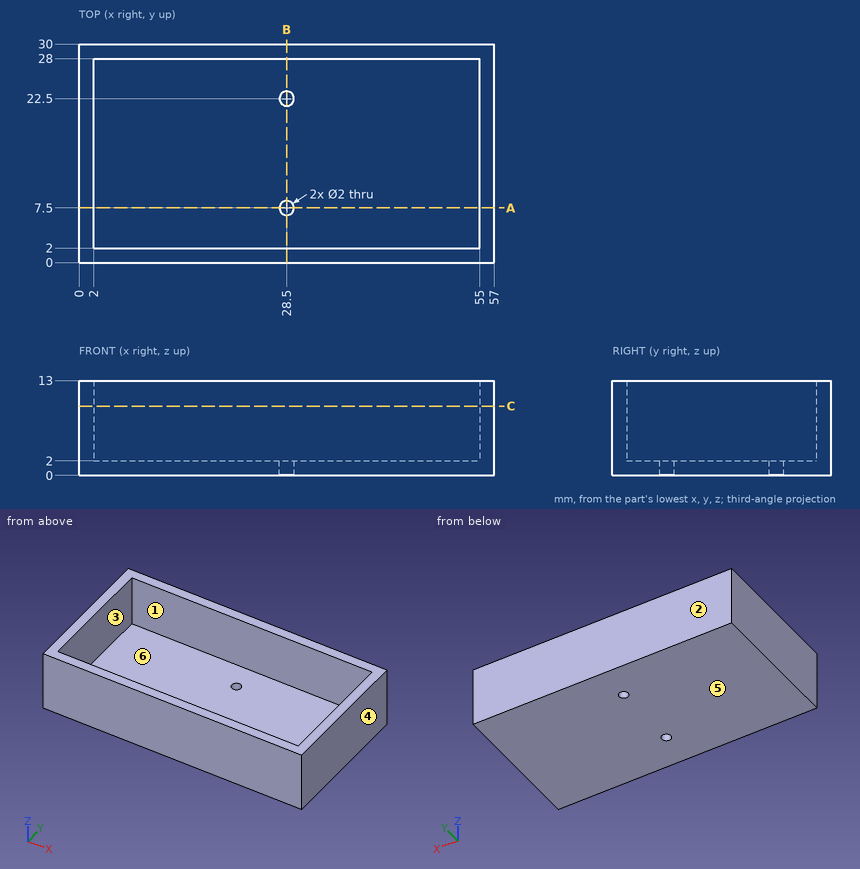
For this review, use the dimensioned drawing (mm, ordinates from the lowest corner) and the shaded views. A direction names the side the tool comes from. Coordinates: 2 decimals unless noted, no trailing zeros. Loops run counter-clockwise (first coordinate to the right, second up) from the corner with the lowest first, then second, coordinate; pieces in that order, holes last. Notation, with made-up numbers: (51, -31.75) - (74, -31.75) arc R12 cw to (74, -15.75) - close; hole circle Ø4 at (83.5, 53.25). An arc over 180 degrees is marked (long way). Use one line per item in the form item = value. Start each with the question number.
1) Take a section at A-A (y = 7.5). State the section outline as (x, z) points.
2) Draft analysis for pull direction X (two halves, no side actions). For the marked faces 1, 2, 3 and 4, state which applies: released by +X, released by -X, zero draft, split by the parting line, or undercut.
3) To check wall thickness, follow probe 1 along Y at (x, z) = (28.5, 1.6); probe 2 along Y at (x, z) = (34, 7.25); probe 3 along X at (y, z) = (27.75, 4.75). State the ranges of each line that lie inside material, in increasing order. Write a range as from..to.
4) Take a section at C-C (z = 9.5). State the section outline as (x, y) points, plus the area to 3 significant figures.
5) Take a section at B-B (x = 28.5). State the section outline as (y, z) points, plus the area to 3 significant figures.
6) For pin 1 (8 mm diameter, centred on x = 35.5, y = 10, fed in from +Z), flat-tipped, find the tip position at first contact; note if it passes through.
7) For the marked faces 5 and 6, list the 3-axis set-ups (+Z, -Z, +X, -X, +Y, -Y) from which the entire face can be reached by the end or side of a thin tool; tool diameter is ignored.
From the geometry:
q1.outline = (0, 0) - (27.5, 0) - (27.5, 2) - (2, 2) - (2, 13) - (0, 13) - close; (29.5, 0) - (57, 0) - (57, 13) - (55, 13) - (55, 2) - (29.5, 2) - close
q2.face_1 = undercut
q2.face_2 = zero draft
q2.face_3 = undercut
q2.face_4 = released by +X
q3.probe_1 = 0..6.5, 8.5..21.5, 23.5..30
q3.probe_2 = 0..2, 28..30
q3.probe_3 = 0..2, 55..57
q4.outline = (0, 0) - (57, 0) - (57, 30) - (0, 30) - close; hole (2, 2) - (55, 2) - (55, 28) - (2, 28) - close
q4.area = 332 mm2
q5.outline = (0, 0) - (6.5, 0) - (6.5, 2) - (2, 2) - (2, 13) - (0, 13) - close; (8.5, 0) - (21.5, 0) - (21.5, 2) - (8.5, 2) - close; (23.5, 0) - (30, 0) - (30, 13) - (28, 13) - (28, 2) - (23.5, 2) - close
q5.area = 96.0 mm2
q6.pin_1 = 2
q7.face_5 = -Z, +X, -X, +Y, -Y
q7.face_6 = +Z
